from build123d import *

# Parameters (mm, degrees)
SKETCH_1_R               = 11
EXTRUDE_1_DEPTH          = 2
SKETCH_2_R               = 1.5
CUT_EXTRUDE_1_DEPTH      = 2
SKETCH_3_R               = 5
EXTRUDE_2_DEPTH          = 10
SKETCH_4_R               = 3
CUT_EXTRUDE_2_DEPTH      = 12
FILLET_1_R               = 0.5
CUT_EXTRUDE_3_REACH      = 21.647
CUT_EXTRUDE_3_END_RADIUS = 5
SKETCH_5_R               = 1.5


with BuildPart() as part:
    # 草图1 → 凸台-拉伸1 (new body)
    with BuildSketch(Plane(origin=(0, 0, 0), x_dir=(1, 0, 0), z_dir=(0, 1, 0))):
        with Locations(Location((0, 0, 0), (0, 0, 270))):
            Circle(SKETCH_1_R)
    extrude(amount=EXTRUDE_1_DEPTH)

    # 草图2 → 切除-拉伸1 (cut)
    with BuildSketch(Plane(origin=(0, 2, 0), x_dir=(1, 0, 0), z_dir=(0, 1, 0))):
        with Locations(Location((0, 8, 0), (0, 0, 270))):
            Circle(SKETCH_2_R)
        with Locations(Location((8, 0, 0), (0, 0, 270))):
            Circle(SKETCH_2_R)
        with Locations(Location((0, -8, 0), (0, 0, 270))):
            Circle(SKETCH_2_R)
        with Locations(Location((-8, 0, 0), (0, 0, 270))):
            Circle(SKETCH_2_R)
    extrude(amount=-CUT_EXTRUDE_1_DEPTH, mode=Mode.SUBTRACT)

    # 草图3 → 凸台-拉伸2 (add)
    with BuildSketch(Plane(origin=(0, 2, 0), x_dir=(1, 0, 0), z_dir=(0, 1, 0))):
        with Locations(Location((0, 0, 0), (0, 0, 270))):
            Circle(SKETCH_3_R)
    extrude(amount=EXTRUDE_2_DEPTH)

    # 草图4 → 切除-拉伸2 (cut)
    with BuildSketch(Plane(origin=(0, 12, 0), x_dir=(1, 0, 0), z_dir=(0, 1, 0))):
        with Locations(Location((0, 0, 0), (0, 0, 270))):
            Circle(SKETCH_4_R)
    extrude(amount=-CUT_EXTRUDE_2_DEPTH, mode=Mode.SUBTRACT)

    # 圆角1
    fillet_1_edges = [part.edges().sort_by_distance(p)[0] for p in [
        (0, 0, -11),
        (0, 12, -5),
        (0, 2, -11),
    ]]
    fillet(fillet_1_edges, radius=FILLET_1_R)

    # 切除-拉伸3: up to this cylinder (the profile starts inside it)
    cut_extrude_3_end = Plane(origin=(0, 7, 0), z_dir=(0, -1, 0)) * Cylinder(CUT_EXTRUDE_3_END_RADIUS, 54.294, mode=Mode.PRIVATE)
    # 草图5 → 切除-拉伸3 (cut, up to the surface)
    with BuildSketch(Plane.XY, mode=Mode.PRIVATE) as cut_extrude_3_sk1:
        with Locations((0, 7)):
            Circle(SKETCH_5_R)
    cut_extrude_3_tool1 = extrude(cut_extrude_3_sk1.sketch, amount=-CUT_EXTRUDE_3_REACH, mode=Mode.PRIVATE) & cut_extrude_3_end
    add(cut_extrude_3_tool1.solids().sort_by_distance((0, 7, 0))[0], mode=Mode.SUBTRACT)


solid = part.part
Verification items for the finished model (mm, model axes). A direction names the side the tool comes from. Round coordinates to 2 decimals unless told otherwise and drop trailing zeros. Loops run counter-clockwise (first coordinate to the right, second up) from the corner with the lowest first, then second, coordinate; pieces in that order, holes last. Notation, with made-up numbers: (20.5, 10.25) - (26.5, 10.25) arc R26 ccw to (26.5, 32.25) - close; hole circle Ø10 at (75.25, 73.25). An arc over 180 degrees is marked (long way). Use one line per item in the form item = value.
1. Section check C-C on y = 7. Record the cut outline in (x, z).
A:
outline = (-1.5, -4.77) - (-1.5, -2.6) arc R3 cw (long way) to (1.5, -2.6) - (1.5, -4.77) arc R5 ccw (long way) to start
2. Section check B-B on x = 0. Give the number of separate pieces and of enclosed holes in the cut face, and give its area (3 significant figures).
A:
separate_pieces = 5
enclosed_holes = 0
area = 53.7 mm²
3. Access from +Z, -Z, +X, -X, +Y, -Y to the whole of each face (thin tool, end or side, straight path). Record for faces 4 (the cylindrical face through (-9.464, 1.014, -0.325)), 5 (the flat face through (-2, 2, 5)).
A:
face_4 = +Y, -Y
face_5 = +Y
4. Draft check along Y on faces 1 (the flat face through (-3, 12, 1)), 2 (the cylindrical face through (1.43, 7.45, -3.78)), 3 (the cylindrical face through (-10.74, 0.99, -2.38)). Enter one of: pulls with the +Y half, pulls with the -Y half, needs draft (parallel to the pull), parting line crosses it, or undercut.
A:
face_1 = pulls with the +Y half
face_2 = undercut
face_3 = needs draft
5. Gauge pin test, flat ends, axial feed: pin 1 Ø3 at (y, z) = (2, 2) entering from +X; pin 2 Ø5 at (x, y) = (0, 7) entering from -Z; pin 3 Ø5 at (x, z) = (8, 0) entering from +Y. Record the tip position at first contact, or that the pin passes through.
A:
pin_1 = 10.98
pin_2 = -5
pin_3 = 2
6. Scan lines: probe 1 along X at (y, z) = (1.2, 0); probe 2 along Y at (x, z) = (-6.5, 4.5); probe 3 along Z at (x, y) = (0.25, 4.25). Record each from-to range of solid material in increasing order.
A:
probe_1 = -11 to -9.5, -6.5 to -3, 3 to 6.5, 9.5 to 11
probe_2 = 0 to 2
probe_3 = -4.99 to -2.99, 2.99 to 4.99
7. Section check A-A on z = 0. Record the cut outline in (x, y), and give its area (3 significant figures).
A:
outline = (-11, 0.5) arc R0.5 ccw to (-10.5, 0) - (-9.5, 0) - (-9.5, 2) - (-10.5, 2) arc R0.5 ccw to (-11, 1.5) - close; (-6.5, 0) - (-3, 0) - (-3, 12) - (-4.5, 12) arc R0.5 ccw to (-5, 11.5) - (-5, 2) - (-6.5, 2) - close; (3, 0) - (6.5, 0) - (6.5, 2) - (5, 2) - (5, 11.5) arc R0.5 ccw to (4.5, 12) - (3, 12) - close; (9.5, 0) - (10.5, 0) arc R0.5 ccw to (11, 0.5) - (11, 1.5) arc R0.5 ccw to (10.5, 2) - (9.5, 2) - close
area = 59.7 mm²
